Could you check a few things on this drawing? It's one solid part, dimensions in mm from its lowest x, y, z. Coordinates: 2 decimals unless noted, no trailing zeros. Write each loop counter-clockwise with the first axis right and the second up, starting at its lowest first coordinate (ties: lowest second). Pieces come first, ordered by that corner, then holes.
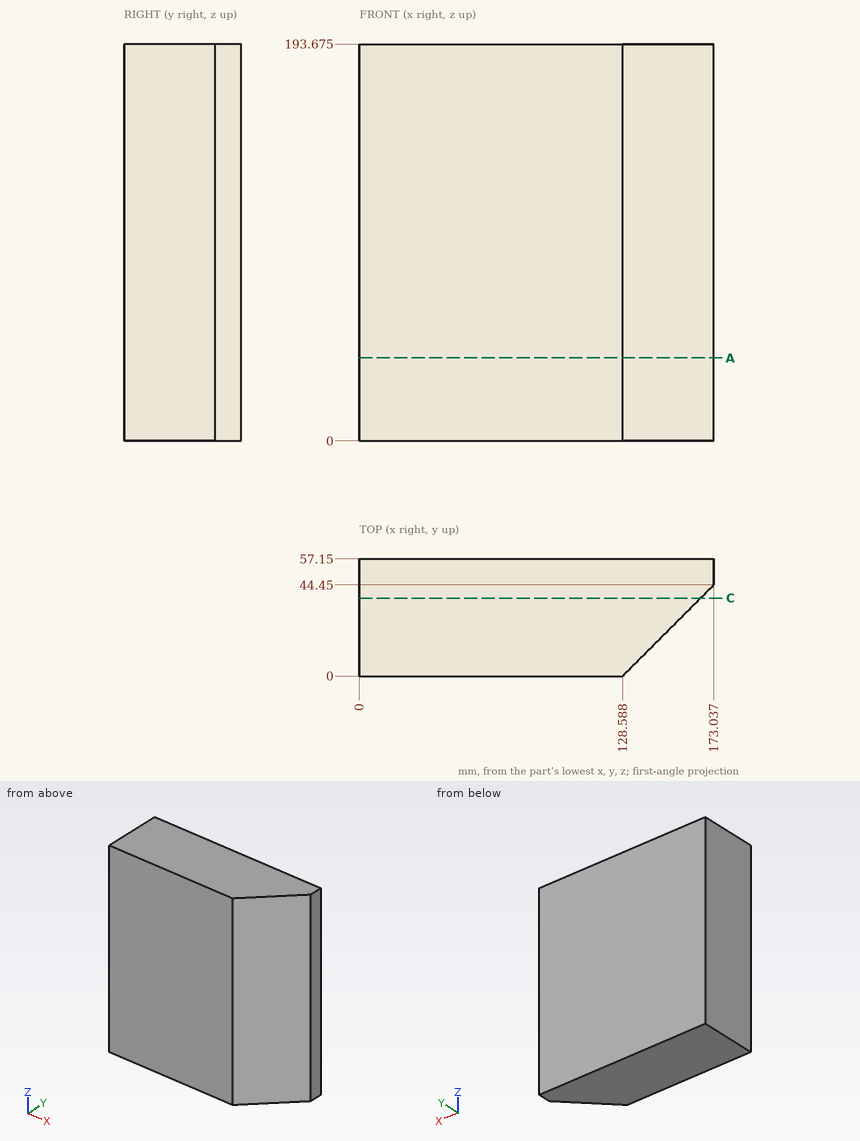
1) Will these pins go through, and if not, where does the flat tip stop? pin 1 (8 mm diameter, centred on y = 7, z = 108.5, fed in from +X); pin 2 (1.5 mm diameter, centred on y = 28, z = 99.5, fed in from +X).
Values follow:
pin 1: stops at x = 139.59
pin 2: stops at x = 157.34
2) Imagine slicing it at A-A on z = 40.5. Please give me the cut outline in (x, y).
Values follow:
outline: (0, 0) - (128.59, 0) - (173.04, 44.45) - (173.04, 57.15) - (0, 57.15) - close
3) I need wall thicknesses on probe 1 along X at (y, z) = (34.5, 150) (1 decimal); probe 2 along X at (y, z) = (41, 105) (1 decimal). Which ranges of each line are inside material? Lowest first, please.
Values follow:
probe 1: x = 0 to 163.1
probe 2: x = 0 to 169.6
4) Imagine slicing it at C-C on y = 38. Please give me the cut outline in (x, z) (1 decimal), then the cut area to 3 significant figures.
Values follow:
outline: (0, 0) - (166.6, 0) - (166.6, 193.7) - (0, 193.7) - close
area: 32,300 mm2
